```python
from build123d import *

# Parameters (mm, degrees)
F2_R     = 4.7625
F3_DEPTH = 9.525
F4_R     = 1.5875
F5_DEPTH = 22.225
F6_R     = 5.08


with BuildPart() as f1:
    # F0 (on Front) → F1 (revolve)
    with BuildSketch(Plane.XZ):
        Polygon((3.81, 1.888357), (31.115, 9.508357), (31.115, 22.208357), (25.902521, 22.208692), (25.902521, 12.683692), (6.905095, 12.683692), (6.985, 22.208357), (6.985, 50.8), (0, 50.8), (0, 1.888357), align=None)
    revolve(axis=Axis((0, 0, 26.344178), (0, 0, -1)))

    # F2 (on face) → F3 (cut)
    with BuildSketch(Plane.XY.offset(50.8)):
        Circle(F2_R)
    extrude(amount=-F3_DEPTH, mode=Mode.SUBTRACT)

    # F4 (on face) → F5 (cut)
    with BuildSketch(Plane(origin=(0, 0, 1.888357), x_dir=(1, 0, 0), z_dir=(0, 0, -1))):
        Circle(F4_R)
    extrude(amount=-F5_DEPTH, mode=Mode.SUBTRACT)

    # F6
    f6_edges = [f1.edges().sort_by_distance(p)[0] for p in [
        (-31.115, 0, 9.508357),
        (-31.115, 0, 22.208357),
        (31.115, 0, 15.858357),
    ]]
    fillet(f6_edges, radius=F6_R)


solid = f1.part
```
Build history of the part. All positions in model axes, mm. A direction names the side the tool comes from. Round coordinates to 2 decimals unless told otherwise and drop trailing zeros. Loops run counter-clockwise (first coordinate to the right, second up) from the corner with the lowest first, then second, coordinate; pieces in that order, holes last.
Item 1: Saw through at A-A (z = 37.5). List the corners of the cut face in (x, y) (3 decimals), then the cut area to 3 significant figures.
Item 2: Drill centre lines: line 1 along Y through (x, z) = (0, 47.75) (1 decimal); line 2 along X through (y, z) = (0, 17) (1 decimal); line 3 along Y through (x, z) = (0, 20). Where is each one in solid material? Low to high.
Item 3: Pin check, flat tips, straight feed: P1, Ø10.5, axis at x = 1, y = 0, coming from the +Z side; P2, Ø1.9, axis at x = 0, y = 0, coming from the +Z side (3 decimals); P3, Ø1.5, axis at x = -2.5, y = -13.5, coming from the +Z side; P4, Ø12, axis at x = 5.5, y = -19.5, coming from the -Z side. Stop position of each tip, or through.
Item 4: Which spindle directions (+Z, -Z, +X, -X, +Y, -Y) get a long thin tool onto all of the face, cutting with end or side? Do faces 1 (the face through (-0.34, 1.55, 12.85)), 2 (the face through (0, 2, 1.888)), 3 (the face through (-0.909, -6.926, 36.704)). Say none if no direction does.
Item 5: Two-plate mould, pull along Z, no slides. Class faces 4 (the face through (0, 0, 24.113)), 5 (the face through (-1.51, 6.78, 17.51)), 6 (the face through (0, 0, 41.275)), 7 (the face through (29.678, -9.346, 15.273)): released by +Z, released by -Z, zero draft, split by the parting line, or undercut.
Worked answers:
1. outline: circle Ø13.97 at (0, 0)
1. area: 153 mm2
2. line 1: y = -7 to -4.8, 4.8 to 7
2. line 2: x = -31.1 to -25.9, -6.9 to -1.6, 1.6 to 6.9, 25.9 to 31.1
2. line 3: y = -30.23 to -25.9, -6.97 to -1.59, 1.59 to 6.97, 25.9 to 30.23
3. P1: stops at z = 50.8
3. P2: stops at z = 41.275
3. P3: stops at z = 12.68
3. P4: stops at z = 4.8
4. face 1: -Z
4. face 2: -Z, +X, -X, +Y, -Y
4. face 3: +Z
5. face 4: released by -Z
5. face 5: undercut
5. face 6: released by +Z
5. face 7: zero draft
